```python
from build123d import *

# Parameters (mm, degrees)
SALIENTE_EXTRUIR1_DEPTH = 20
REDONDEO1_R             = 10
SALIENTE_EXTRUIR2_START = 20
CROQUIS1_4_R            = 4.5
SALIENTE_EXTRUIR2_DEPTH = 20
SALIENTE_EXTRUIR4_DEPTH = 5
REDONDEO4_R             = 5
REDONDEO5_R             = 2


with BuildPart() as part:
    # Croquis1 → Saliente-Extruir1 (new body)
    with BuildSketch(Plane(origin=(0, 0, 0), x_dir=(1, 0, 0), z_dir=(0, 1, 0))):
        with BuildLine():
            Line((4.71210557073282, 8.494038111608782), (2.980054763163943, 7.494038111608782))
            ThreePointArc((2.9800547631639436, 7.494038111608781), (6.495190528383288, 3.749999999999996), (7.9800547631639365, -1.1662159262356018))
            Line((7.980054763163938, -1.166215926235604), (16.640308801008324, 3.8337840737643942))
            Line((16.640308801008324, 3.833784073764395), (11.640308801008324, 12.49403811160878))
            ThreePointArc((11.640308801008327, 12.494038111608782), (7.486283619207324, 17.729429010253995), (1.992335720896067, 21.53492235058391))
            ThreePointArc((1.9923357208960657, 21.534922350583905), (-4.3821884132033615, 18.52294902668032), (2.49e-15, 13))
            ThreePointArc((4.3e-16, 13), (3.259893842188938, 11.692210023771297), (4.712105570732819, 8.494038111608784))
        make_face()
    extrude(amount=-SALIENTE_EXTRUIR1_DEPTH)

    # Redondeo1
    redondeo1_edges = [part.edges().sort_by_distance(p)[0] for p in [
        (16.640308801008324, -10, -3.8337840737643947),
    ]]
    fillet(redondeo1_edges, radius=REDONDEO1_R - 0.0001)  # a hair under: the kernel refuses the full size

    # Croquis1<4> → Saliente-Extruir2 (add)
    with BuildSketch(Plane(origin=(0, 0, 0), x_dir=(1, 0, 0), z_dir=(0, 1, 0)).offset(SALIENTE_EXTRUIR2_START)):
        with Locations(Location((4e-17, 17.5, 0), (0, 0, 270))):
            Circle(CROQUIS1_4_R)
    extrude(amount=-SALIENTE_EXTRUIR2_DEPTH)

    # Croquis2 → Saliente-Extruir4 (add)
    with BuildSketch(Plane(origin=(0, 0, 0), x_dir=(1, 0, 0), z_dir=(0, 1, 0))):
        with BuildLine():
            ThreePointArc((9.051706443450353, 26.551706443450232), (1.1156846733798031, 30.2523341701189), (-7.342378354819137, 27.986003012181577))
            ThreePointArc((-7.342378354819137, 27.986003012181577), (-8.36164556563995, 22.20545141012103), (-2.581093963579654, 21.186184199300502))
            ThreePointArc((-2.581093963579654, 21.186184199300502), (0.3922008423644143, 21.98287614141279), (3.181980515339327, 20.681980515339635))
            ThreePointArc((3.181980515339327, 20.681980515339635), (9.051706443449934, 20.681980515339355), (9.051706443450353, 26.551706443450232))
        make_face()
        with BuildLine():
            ThreePointArc((7.531057041767888, 25.031057041767813), (0.928254243367484, 28.109994551949146), (-6.108889031901341, 26.224397694318867))
            ThreePointArc((-6.108889031901341, 26.224397694318867), (-6.600040247777167, 23.438940733039082), (-3.814583286497142, 22.947789517162914))
            ThreePointArc((-3.814583286497142, 22.947789517162914), (0.579631272376833, 24.12521575958216), (4.702629917021658, 22.20262991702166))
            ThreePointArc((4.702629917021658, 22.20262991702166), (7.531057041767845, 22.20262991702162), (7.531057041767888, 25.031057041767813))
        make_face(mode=Mode.SUBTRACT)
    extrude(amount=-SALIENTE_EXTRUIR4_DEPTH)

    # Redondeo4
    redondeo4_edges = [part.edges().sort_by_distance(p)[0] for p in [
        (5.278570690107173, -2.5, -19.551853938657132),
        (-2.5810939635796544, -2.5, -21.1861841993005),
    ]]
    fillet(redondeo4_edges, radius=REDONDEO4_R)

    # Redondeo5
    redondeo5_edges = [part.edges().sort_by_distance(p)[0] for p in [
        (4.712105570732819, -10, -8.494038111608784),
    ]]
    fillet(redondeo5_edges, radius=REDONDEO5_R)


solid = part.part
```
Geometry check sheet. Reference: the model listing, model coordinates, mm. A direction names the side the tool comes from. Round coordinates to 2 decimals unless told otherwise and drop trailing zeros. Order: outer loops, then holes, each group sorted by start corner. A loop starts at its lowest first (then second) coordinate and runs counter-clockwise, first axis right, second up. Notation, with made-up numbers: (33.5, 8.5) -> (68.5, 8.5) arc R23 cw to (68.5, 35.5) -> close; hole circle Ø2 at (-16, -30). An arc over 180 degrees is marked (long way). Return JSON: item names as keys, results as strings. Group by question number.
Q1. Section check A-A, the plane x = 5.5. Record the boundary of the cut face in (y, z), plus the area to 3 significant figures.
Q2. Section check D-D, the plane y = 14.5. Record the boundary of the cut face in (x, z), plus the area to 3 significant figures.
Q3. Tool access check on faces 4 (the cylindrical face through (1.03, -2.46, -28.1)), 5 (the cylindrical face through (4.343, -10.14, -8.889)). Record the directions out of +Z, -Z, +X, -X, +Y, -Y that give a thin tool (end or side, any length) a straight path to the whole face; none if there is none.
Q4. Section check C-C, the plane z = -11. Record the boundary of the cut face in (x, y).
Q5. Release check for a two-part mould opening along Z. For faces 1 (the cylindrical face through (2.46, -9.86, -12.31)), 2 (the cylindrical face through (-4.39, 4.72, -18.48)), 3 (the flat face through (5, 0, -16)) record: released by +Z, released by -Z, zero draft, split by the parting line, or undercut.
Q6. Material ranges on probe 1 along Y at (x, z) = (8, -15); probe 2 along Y at (x, z) = (6, -26.5); probe 3 along Z at (x, y) = (0, 13.5), recorded low to high. Write a range as from..to.
Numbers:
{
 "1": {"outline": "(-20, -19.39) -> (-5, -19.39) -> (-5, -21.71) -> (0, -21.71) -> (0, -5.2) -> (-20, -5.2) -> close; (-5, -29.06) -> (0, -29.06) -> (0, -26.62) -> (-5, -26.62) -> close", "area": "308 mm^2"},
 "2": {"outline": "circle Ø9 at (0, -17.5)", "area": "63.6 mm^2"},
 "3": {"face 4": "+Y, -Y", "face 5": "-X, +Y, -Y"},
 "4": {"outline": "(3.86, -20) -> (12.35, -20) -> (12.35, 0) -> (3.86, 0) -> close"},
 "5": {"face 1": "undercut", "face 2": "split by the parting line", "face 3": "zero draft"},
 "6": {"probe 1": "-20..0", "probe 2": "-5..0", "probe 3": "-22..-13"}
}
